Autodesk Inventor part; units mm, degrees
ref_plane "Work Plane1" through (-30.997, 0, 0) normal (0, -0.8660254, -0.5) x (1, 0, 0)
ref_plane "YZ Plane" through (0, 0, 0) normal (1, 0, 0) x (0, 1, 0)
ref_plane "XZ Plane" through (0, 0, 0) normal (0, 1, 0) x (-1, 0, 0)
sketch "Sketch1" plane through (0, 0, 0) normal (1, 0, 0) x (0, 1, 0)
  line L0 (-17.3205, 0) -> (-8.6603, 15)
  line L1 (-8.6603, 15) -> (8.6603, 15)
  line L2 (8.6603, 15) -> (17.3205, 0)
  line L3 (17.3205, 0) -> (8.6603, -15)
  line L4 (8.6603, -15) -> (-8.6603, -15)
  line L5 (-8.6603, -15) -> (-17.3205, 0)
  point P0 (0, 0)
  point P1 (0, 0)
  dimension "d0" = 34.641
extrude "Body" add sketch "Sketch1" along normal blind 19
sketch "Sketch2" plane through (0, 0, 0) normal (0, 0, 1) x (1, 0, 0)
  line L0 (0, 8.6603) -> (0, 17.3205)
  line L1 (0, 17.3205) -> (19, 17.3205)
  line L2 (19, 8.6603) -> (19, 17.3205)
  line L3 (-3.8, 0) -> (22.8, 0)
  line L4 (2.0037, 17.3205) -> (0, 13.85)
  line L5 (16.9963, 17.3205) -> (19, 13.85)
  dimension "d3" = 30
  dimension "d4" = 30
  dimension "d5" = 27.7
  dimension "d6" = 27.7
revolve "Chamfer1" cut sketch "Sketch2" angle 360 about axis through (-10, 0, 0) along (1, 0, 0)
sketch "Sketch3" plane through (19, 0, 0) normal (1, 0, 0) x (0, 0, -1)
  arc A0 (-0.625, -1.0825) -> (0.625, -1.0825) centre (0, 0) ccw
hole "Thread" at (19, 0, 0) direction (-1, 0, 0) diameter 17.294 end through all
chamfer "Chamfer2" distance 1.3532 angle 30 1 edges at (19, 0, 8.647) measured on face at (19, 11.9605, -1.4523)
chamfer "Chamfer3" distance 1.3532 angle 30 1 edges at (0, 0, 8.647) measured on face at (0, 11.9605, -1.4523)
ref_plane "Work Plane1" through (-30.997, 0, 0) normal (0, -0.8660254, -0.5) x (1, 0, 0)
equation "\"d0\" = 1.1547 * SW"
equation "\"d1\" = KOH"
equation "\"d3\" = ANG1"
equation "\"d4\" = ANG2"
equation "\"d5\" = SW0"
equation "\"d6\" = SW01"
equation "\"d8\" = -0.5 * GD1 + 0.5 * NND"
equation "\"d40\" = -0.5 * GD1 + 0.5 * NND"
equation "\"d10\" = -0.5 * GD1 + 0.5 * NND"
equation "\"d41\" = -0.5 * GD1 + 0.5 * NND"
equation "\"ANG1\" = 30deg"
equation "\"ANG2\" = 30deg"
equation "\"KOH\" = 19"
equation "\"SW0\" = 27.7"
equation "\"SW01\" = SW0"
equation "\"GUL\" = 0.541266 * PTC"
equation "\"TOA\" = 30deg"
equation "\"PTC\" = 2.5"
equation "\"E0\" = 1.155 * SW"
equation "\"GAL\" = 0.541266 * PTC"
properties part number "ISO 4034 - M20" material "Steel"
Could you check a few things on this model? Use its own coordinates, in mm. Give positions to 0.01 mm unless a question says otherwise; leave off trailing zeros. Order: outer loops, then holes, each group sorted by start corner. A loop starts at its lowest first (then second) coordinate and runs counter-clockwise, first axis right, second up.
Item 1: If we mould it in two halves opening along Y, with no side actions, what happens to faces 1 (the face through (9.376, -12.93, -7.605)), 2 (the face through (9, 0, 15)), 3 (the face through (9.378, 5.262, 6.862)), 4 (the face through (0.125, -11.163, -8.56))? For each: pulls with the +Y half, pulls with the -Y half, needs draft (parallel to the pull), parting line crosses it, or undercut.
Item 2: If we section it at A-A, the plane y = 0: Write out the boundary of the cut face in (x, z).
Item 3: I'm going to push flat-ended pins straight in: pin 1 (8 mm diameter, centred on x = 12.5, z = 1, fed in from +Y); pin 2 (1 mm diameter, centred on x = 12.5, z = 9, fed in from +Y); pin 3 (5 mm diameter, centred on x = 8, z = -5.5, fed in from +Y). Where does each tip first touch, or does it pass through?
Item 4: If we section it at B-B, the plane x = 12: Write out the boundary of the cut face in (y, z), plus the area to 3 significant figures.
Item 5: I need wall thicknesses on line 1 (Z direction, x = 6.5, y = 0); line 2 (Y direction, x = 11.25, z = 0); line 3 (Y direction, x = 5, z = -1.75). Which ranges of each line are inside material? Lowest first, please.
Values:
1. face 1: pulls with the -Y half
1. face 2: needs draft
1. face 3: undercut
1. face 4: parting line crosses it
2. outline: (0, -13.85) - (0.66, -15) - (18.34, -15) - (19, -13.85) - (19, -10) - (18.22, -8.65) - (0.78, -8.65) - (0, -10) - close; (0, 10) - (0.78, 8.65) - (18.22, 8.65) - (19, 10) - (19, 13.85) - (18.34, 15) - (0.66, 15) - (0, 13.85) - close
3. pin 1: stops at y = 17.32
3. pin 2: stops at y = 12.41
3. pin 3: stops at y = 15.59
4. outline: (-17.32, 0) - (-8.66, -15) - (8.66, -15) - (17.32, 0) - (8.66, 15) - (-8.66, 15) - close; hole circle Ø17.29 at (0, 0)
4. area: 545 mm2
5. line 1: z = -15 to -8.65, 8.65 to 15
5. line 2: y = -17.32 to -8.65, 8.65 to 17.32
5. line 3: y = -16.31 to -8.47, 8.47 to 16.31
